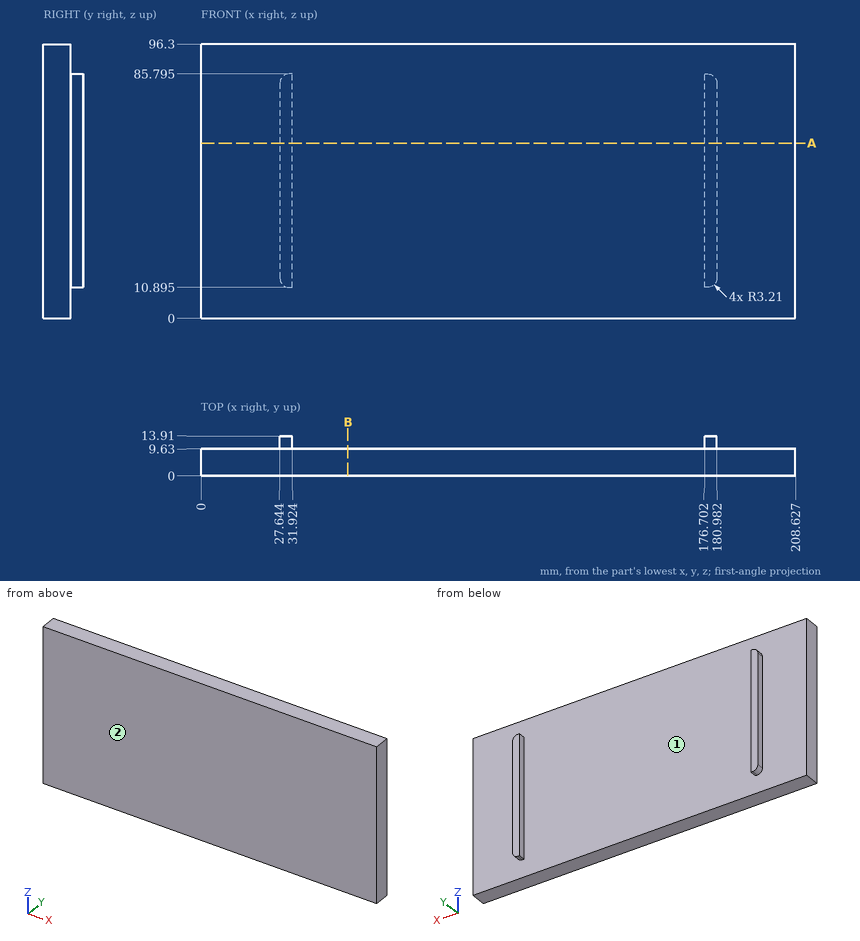
Can you work these out from the drawing? Everything is in mm from the part's minimum corner. Give positions to 0.01 mm unless a question says otherwise; leave off trailing zeros. Loops run counter-clockwise (first coordinate to the right, second up) from the corner with the lowest first, then second, coordinate; pieces in that order, holes last. Notation, with made-up numbers: (25, 10) -> (52, 10) arc R18 cw to (52, 33) -> close; hole circle Ø11 at (-36.75, 69). An arc over 180 degrees is marked (long way). Return JSON: item names as keys, results as strings.
Q1. I need wall thicknesses on probe 1 along X at (y, z) = (11.75, 29.5) (1 decimal); probe 2 along Y at (x, z) = (65, 17); probe 3 along X at (y, z) = (12.5, 85) (1 decimal). Which ranges of each line are inside material? Lowest first, please.
Checks:
{"probe 1": "x = 27.6 to 31.9, 176.7 to 181", "probe 2": "y = 0 to 9.63", "probe 3": "x = 28.7 to 31.9, 176.7 to 179.9"}
Q2. I want a section at A-A, the plane z = 61.5. List the corners of the cut face in (x, y) for me (1 decimal), then the cut area to 3 significant figures.
Checks:
{"outline": "(0, 0) -> (208.6, 0) -> (208.6, 9.6) -> (181, 9.6) -> (181, 13.9) -> (176.7, 13.9) -> (176.7, 9.6) -> (31.9, 9.6) -> (31.9, 13.9) -> (27.6, 13.9) -> (27.6, 9.6) -> (0, 9.6) -> close", "area": "2,050 mm2"}
Q3. We'd pull the mould along X, two halves only. Please class the marked faces 1 and 2: released by +X, released by -X, zero draft, split by the parting line, or undercut.
Checks:
{"face 1": "undercut", "face 2": "zero draft"}
Q4. For pin 1 Ø1.2 at (x, y) = (177.5, 12) entering from +Z (1 decimal); pin 2 Ø3 at (x, y) = (89, 10.5) entering from +Z; pin 3 Ø1.2 at (x, y) = (31.5, 11) entering from -Z (1 decimal); pin 4 Ø2 at (y, z) = (12.5, 32.5) entering from +X, each with a flat end and sliding along its axis, tell me the tip position at first contact or that it passes through.
Checks:
{"pin 1": "stops at z = 85.8", "pin 2": "stops at z = 96.3", "pin 3": "stops at z = 10.9", "pin 4": "stops at x = 180.98"}
Q5. I want a section at B-B, the plane x = 51.5. List the corners of the cut face in (y, z) for me.
Checks:
{"outline": "(0, 0) -> (9.63, 0) -> (9.63, 96.3) -> (0, 96.3) -> close"}
